```python
from build123d import *

# Parameters (mm, degrees)
ESBO_O1_W                = 120
ESBO_O1_H                = 40
ESBO_O1_R                = 2.25
RESSALTO_EXTRUS_O1_DEPTH = 28
ESBO_O2_W                = 10
ESBO_O2_H                = 40
CORTE_EXTRUS_O1_DEPTH    = 30
FILETE1_R                = 20
FILETE2_R                = 5
ESBO_O3_R                = 2.5
CORTE_EXTRUS_O2_DEPTH    = 40


with BuildPart() as part:
    # Esboço1 → Ressalto-extrusão1 (new body)
    with BuildSketch(Plane.XY):
        with Locations((60, 20)):
            Rectangle(ESBO_O1_W, ESBO_O1_H)
        with Locations((10, 20)):
            Circle(ESBO_O1_R, mode=Mode.SUBTRACT)
    extrude(amount=RESSALTO_EXTRUS_O1_DEPTH)

    # Esboço2 → Corte-extrusão1 (cut)
    with BuildSketch(Plane(origin=(120, 0, 0), x_dir=(0, 0, -1), z_dir=(1, 0, 0))):
        with Locations((-14, 20)):
            Rectangle(ESBO_O2_W, ESBO_O2_H)
    extrude(amount=-CORTE_EXTRUS_O1_DEPTH, mode=Mode.SUBTRACT)

    # Filete1
    filete1_edges = [part.edges().sort_by_distance(p)[0] for p in [
        (0, 0, 14),
        (0, 40, 14),
    ]]
    fillet(filete1_edges, radius=FILETE1_R - 0.0001)  # a hair under: the kernel refuses the full size

    # Filete2
    filete2_edges = [part.edges().sort_by_distance(p)[0] for p in [
        (69.99995, 40, 28),
        (69.99995, 0, 28),
        (69.99995, 0, 0),
        (5.857835087, 34.142164913, 0),
        (5.857835087, 5.857835087, 0),
        (5.857835087, 34.142164913, 28),
        (5.857835087, 5.857835087, 28),
        (69.99995, 40, 0),
    ]]
    fillet(filete2_edges, radius=FILETE2_R)

    # Esboço3 → Corte-extrusão2 (cut)
    with BuildSketch(Plane.XY.offset(28)):
        with Locations((105, 20)):
            Circle(ESBO_O3_R)
    extrude(amount=-CORTE_EXTRUS_O2_DEPTH, mode=Mode.SUBTRACT)


solid = part.part
```
The model under review builds one solid part; all positions refer to its coordinate system, in mm. A direction names the side the tool comes from. Round coordinates to 2 decimals unless told otherwise and drop trailing zeros. Loops run counter-clockwise (first coordinate to the right, second up) from the corner with the lowest first, then second, coordinate; pieces in that order, holes last.
Item 1: Take a section at C-C (z = 21.25). Give the number of separate pieces and of enclosed holes in the cut face, then the cut area to 3 significant figures.
Determined:
separate pieces: 1
enclosed holes: 2
area: 4,590 mm2
Item 2: Clearance check with flat-ended pins moving along their axes: pin 1 Ø1.5 at (y, z) = (20, 11) entering from +X; pin 2 Ø1.5 at (y, z) = (32, 12) entering from -X. State where each tip first meets the part, or that it passes through.
Determined:
pin 1: stops at x = 90
pin 2: stops at x = 3.46
Item 3: For faces 4 (the face through (109, 20, 19)), 5 (the face through (69, 2, 27)), list the 3-axis set-ups (+Z, -Z, +X, -X, +Y, -Y) from which the entire face can be reached by the end or side of a thin tool; tool diameter is ignored.
Determined:
face 4: +X, +Y, -Y
face 5: +Z, +X, -X, -Y
Item 4: Take a section at A-A (x = 97.5). Write out the cut boundary in (y, z), then the cut area to 3 significant figures.
Determined:
outline: (0, 5) arc R5 ccw to (5, 0) - (35, 0) arc R5 ccw to (40, 5) - (40, 9) - (0, 9) - close; (0, 19) - (40, 19) - (40, 23) arc R5 ccw to (35, 28) - (5, 28) arc R5 ccw to (0, 23) - close
area: 699 mm2
Item 5: For line 1 (Z direction, x = 94.5, y = 10); line 2 (X direction, y = 19.5, z = 19.5); line 3 (Y direction, x = 105, z = 21.5), list the stretches that pass through material, from the lowest coordinate up.
Determined:
line 1: z = 0 to 9, 19 to 28
line 2: x = 0.01 to 7.81, 12.19 to 102.55, 107.45 to 120
line 3: y = 0 to 17.5, 22.5 to 40
Item 6: Mouldability with a two-part tool opening along X and no side actions: class faces 1 (the face through (120, 20, 23)), 2 (the face through (9.512, 17.804, 13.804)), 3 (the face through (109, 20, 9)) as released by +X, released by -X, zero draft, split by the parting line, or undercut.
Determined:
face 1: released by +X
face 2: undercut
face 3: zero draft
Item 7: Take a section at D-D (x = 23.5). Write out the cut boundary in (y, z).
Determined:
outline: (0, 5) arc R5 ccw to (5, 0) - (35, 0) arc R5 ccw to (40, 5) - (40, 23) arc R5 ccw to (35, 28) - (5, 28) arc R5 ccw to (0, 23) - close
